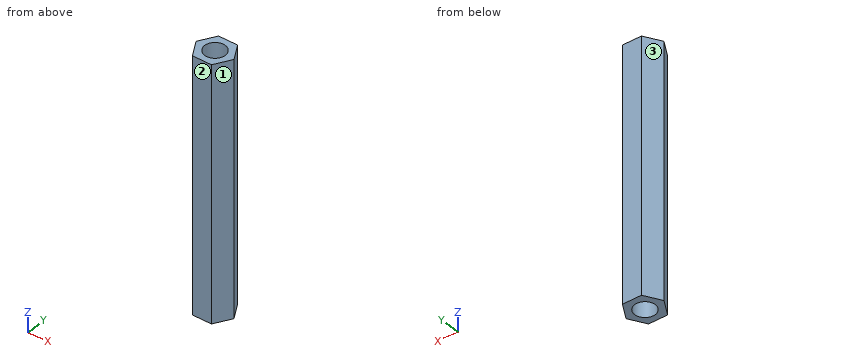
Autodesk Inventor part; units mm, degrees
ref_plane "YZ Plane" through (0, 0, 0) normal (1, 0, 0) x (0, 1, 0)
ref_plane "XZ Plane" through (0, 0, 0) normal (0, 1, 0) x (-1, 0, 0)
ref_plane "XY Plane" through (0, 0, 0) normal (0, 0, 1) x (1, 0, 0)
sketch "Base" plane through (0, 0, 0) normal (0, 0, 1) x (1, 0, 0)
  circle A0 centre (0, 0) radius 1.5 construction
  circle A1 centre (0, 0) radius 2.25 construction
  line L0 (1.125, 1.9486) -> (2.25, 0)
  line L1 (2.25, 0) -> (1.125, -1.9486)
  line L2 (1.125, -1.9486) -> (-1.125, -1.9486)
  line L3 (-1.125, -1.9486) -> (-2.25, 0)
  line L4 (-2.25, 0) -> (-1.125, 1.9486)
  line L5 (-1.125, 1.9486) -> (1.125, 1.9486)
  line L6 (-3.15, 0) -> (3.15, 0)
  dimension "d1" = 4.5
  dimension "d0" = 3
extrude "BaseFeature" add sketch "Base" along normal blind 30
sketch "MountHole" plane through (0, 0, 30) normal (0, 0, 1) x (1, 0, 0)
  point P0 (0, 0)
hole "MountHoleFeature" at (0, 0, 30) direction (0, 0, -1) diameter 2.459 end through all
properties part number "M3-Standoff-30mm"
The listing builds one solid part. Answer for the finished solid, in the listing's coordinates (mm). Face numbers are marked on the shaded views. Coordinates: 2 decimals unless noted, no trailing zeros. Write each loop counter-clockwise with the first axis right and the second up, starting at its lowest first coordinate (ties: lowest second). Pieces come first, ordered by that corner, then holes. Notation, with made-up numbers: M -9,69 L 40,69 A15 ccw 40,73 Z; hole C 11.5,3 d4. An arc over 180 degrees is marked long. Use one line per item in the form item = value.
Item 1: Given P1, Ø1.5, axis at y = -1.5, z = 12, coming from the -X side, flat-ended and moving along its own axis, determine where the tip first touches the part or whether it passes through.
Model answer:
P1 = -1.82
Item 2: Find section D-D, the plane x = -1.7. Give the vertices of the cut face in (y, z).
Model answer:
outline = M -0.95,0 L 0.95,0 L 0.95,30 L -0.95,30 Z
Item 3: The mould has two halves that part along X. Classify the marked faces 1, 2 and 3: released by +X, released by -X, zero draft, split by the parting line, or undercut.
Model answer:
face_1 = released by +X
face_2 = zero draft
face_3 = released by -X
Item 4: Find section C-C, the plane y = -0.9. Give the vertices of the cut face in (x, z), plus the area to 3 significant figures.
Model answer:
outline = M -1.73,0 L -0.84,0 L -0.84,30 L -1.73,30 Z; M 0.84,0 L 1.73,0 L 1.73,30 L 0.84,30 Z
area = 53.6 mm2
Item 5: Find the intervals of material crossed by probe 1 along Y at (x, z) = (0, 12.5); probe 2 along X at (y, z) = (0.8, 9.25); probe 3 along X at (y, z) = (0.55, 20.25), in increasing order.
Model answer:
probe_1 = -1.95 to -1.23, 1.23 to 1.95
probe_2 = -1.79 to -0.93, 0.93 to 1.79
probe_3 = -1.93 to -1.1, 1.1 to 1.93
Item 6: Find section A-A, the plane x = 0. Give the vertices of the cut face in (y, z).
Model answer:
outline = M -1.95,0 L -1.23,0 L -1.23,30 L -1.95,30 Z; M 1.23,0 L 1.95,0 L 1.95,30 L 1.23,30 Z
